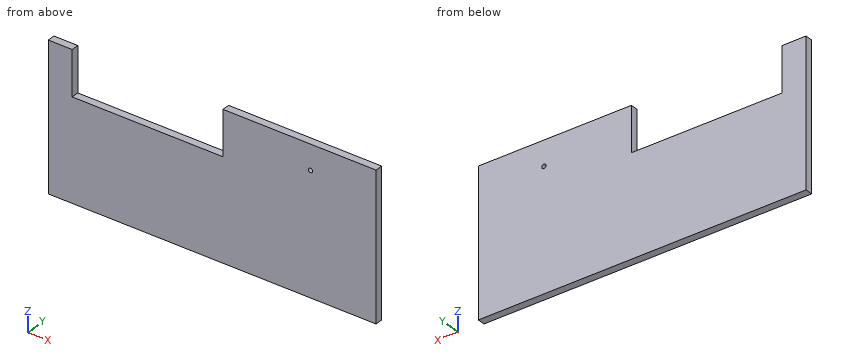
```python
from build123d import *

# Parameters (mm, degrees)
BOSS_EXTRUDE1_DEPTH = 3
SKETCH2_R           = 0.85
CUT_EXTRUDE1_DEPTH  = 143.920705638


with BuildPart() as part:
    # Sketch1 → Boss-Extrude1 (new body)
    with BuildSketch(Plane(origin=(0, 0, 0), x_dir=(1, 0, 0), z_dir=(0, 1, 0))):
        Polygon((130.41, 0), (0, 0), (0, -58.4), (9.5, -58.4), (9.5, -40.4), (69.5, -40.4), (69.5, -58.4), (130.41, -58.4), align=None)
    extrude(amount=BOSS_EXTRUDE1_DEPTH)

    # Sketch2 → Cut-Extrude1 (cut, through all)
    with BuildSketch(Plane(origin=(0, 3, 0), x_dir=(1, 0, 0), z_dir=(0, 1, 0))):
        with Locations(Location((104.3, -48.4, 0), (0, 0, 270))):
            Circle(SKETCH2_R)
    extrude(amount=-CUT_EXTRUDE1_DEPTH, mode=Mode.SUBTRACT)


solid = part.part
```
Model file for the job. Use its own axes, mm. Give positions to 0.01 mm unless a question says otherwise; leave off trailing zeros. Order: outer loops, then holes, each group sorted by start corner. A loop starts at its lowest first (then second) coordinate and runs counter-clockwise, first axis right, second up.
1) Pin check, flat tips, straight feed: pin 1 (2 mm diameter, centred on x = 104.3, z = 48.4, fed in from +Y); pin 2 (0.9 mm diameter, centred on x = 50, y = 2, fed in from +Z). Stop position of each tip, or through.
2) Saw through at B-B, the plane x = 50. Write the cut outline in (y, z), then the cut area to 3 significant figures.
3) Wall check: probe 1 along X at (y, z) = (2.3, 48.4); probe 2 along Z at (x, y) = (104.3, 0.7); probe 3 along Z at (x, y) = (38.5, 0.4). Give the ranges that are in metal, low to high.
4) Saw through at A-A, the plane y = 1.65. Write the cut outline in (x, z).
Computed:
1. pin 1: stops at y = 3
1. pin 2: stops at z = 40.4
2. outline: (0, 0) - (3, 0) - (3, 40.4) - (0, 40.4) - close
2. area: 121 mm2
3. probe 1: x = 0 to 9.5, 69.5 to 103.45, 105.15 to 130.41
3. probe 2: z = 0 to 47.55, 49.25 to 58.4
3. probe 3: z = 0 to 40.4
4. outline: (0, 0) - (130.41, 0) - (130.41, 58.4) - (69.5, 58.4) - (69.5, 40.4) - (9.5, 40.4) - (9.5, 58.4) - (0, 58.4) - close; hole circle Ø1.7 at (104.3, 48.4)
